Verification items for the finished model (mm, model axes). A direction names the side the tool comes from. Give positions to 0.01 mm unless a question says otherwise; leave off trailing zeros. Loops run counter-clockwise (first coordinate to the right, second up) from the corner with the lowest first, then second, coordinate; pieces in that order, holes last. Notation, with made-up numbers: (58, -26.5) - (101, -26.5) arc R15 cw to (101, 2.5) - close; hole circle Ø2 at (87.25, -28.75). An arc over 180 degrees is marked (long way). Use one line per item in the form item = value.
```python
from build123d import *

# Parameters (mm, degrees)
SKETCH1_W           = 5.6
SKETCH1_H           = 5.6
BOSS_EXTRUDE1_DEPTH = 1
SKETCH1_3_R         = 1.85
BOSS_EXTRUDE2_DEPTH = 11.7
SKETCH2_R           = 0.6
CUT_EXTRUDE1_DEPTH  = 5
BOSS_EXTRUDE3_START = 2
SKETCH3_R           = 2.25
SKETCH3_R_2         = 0.6
BOSS_EXTRUDE3_DEPTH = 2
CHAMFER1_SIZE       = 1.5
CHAMFER1_SIZE2      = 0.401923789
SKETCH4_W           = 1
SKETCH4_H           = 5.286883196
CUT_EXTRUDE3_DEPTH  = 4
FILLET1_R           = 1.5


with BuildPart() as part:
    # Sketch1 → Boss-Extrude1 (new body)
    with BuildSketch(Plane.XY):
        Rectangle(SKETCH1_W, SKETCH1_H)
    extrude(amount=BOSS_EXTRUDE1_DEPTH)

    # Sketch1<3> → Boss-Extrude2 (add)
    with BuildSketch(Plane.XY):
        Circle(SKETCH1_3_R)
    extrude(amount=-BOSS_EXTRUDE2_DEPTH)

    # Sketch2 → Cut-Extrude1 (cut)
    with BuildSketch(Plane(origin=(0, 0, -11.7), x_dir=(-1, 0, 0), z_dir=(0, 0, -1))):
        Circle(SKETCH2_R)
    extrude(amount=-CUT_EXTRUDE1_DEPTH, mode=Mode.SUBTRACT)

    # Sketch3 → Boss-Extrude3 (add)
    with BuildSketch(Plane(origin=(0, 0, -11.7), x_dir=(-1, 0, 0), z_dir=(0, 0, -1)).offset(BOSS_EXTRUDE3_START)):
        Circle(SKETCH3_R)
        Circle(SKETCH3_R_2, mode=Mode.SUBTRACT)
    extrude(amount=-BOSS_EXTRUDE3_DEPTH)

    # Chamfer1
    chamfer1_edges = [part.edges().sort_by_distance(p)[0] for p in [
        (2.25, 0, -13.7),
    ]]
    chamfer1_side = [part.faces().sort_by_distance(p)[0] for p in [
        (2.25, 0, -12.7),
    ]]
    chamfer(chamfer1_edges, length=CHAMFER1_SIZE, length2=CHAMFER1_SIZE2, reference=chamfer1_side[0])

    # Sketch4 → Cut-Extrude3 (cut)
    with BuildSketch(Plane(origin=(0, 0, -13.7), x_dir=(-1, 0, 0), z_dir=(0, 0, -1))):
        Rectangle(SKETCH4_W, SKETCH4_H)
    extrude(amount=-CUT_EXTRUDE3_DEPTH, mode=Mode.SUBTRACT)

    # Fillet1
    fillet1_edges = [part.edges().sort_by_distance(p)[0] for p in [
        (2.25, 0, -12.2),
        (-2.25, 0, -12.2),
    ]]
    fillet(fillet1_edges, radius=FILLET1_R)


solid = part.part
```
1. Section check A-A, the plane x = 0. Record the cut outline in (y, z).
Result set:
outline = (-2.8, 0) - (-1.85, 0) - (-1.85, -9.7) - (-0.6, -9.7) - (-0.6, -6.7) - (0.6, -6.7) - (0.6, -9.7) - (1.85, -9.7) - (1.85, 0) - (2.8, 0) - (2.8, 1) - (-2.8, 1) - close
2. Section check C-C, the plane y = 2.5. Record the cut outline in (x, z), then the cut area to 3 significant figures.
Result set:
outline = (-2.8, 0) - (2.8, 0) - (2.8, 1) - (-2.8, 1) - close
area = 5.60 mm²
3. Depth check by flat-ended pin: pin 1 Ø2 at (y, z) = (-1, -11) entering from +X; pin 2 Ø1 at (y, z) = (0, -6.5) entering from +X; pin 3 Ø1.5 at (x, z) = (0, -1.5) entering from -Y. Enter the tip coordinate at first touch or a pass-through.
Result set:
pin_1 = 2.23
pin_2 = 1.85
pin_3 = -1.85
4. Section check D-D, the plane z = -1.5. Record the cut outline in (x, y).
Result set:
outline = circle Ø3.7 at (0, 0)
5. Scan lines: probe 1 along Y at (x, z) = (0, -9.5); probe 2 along Z at (x, y) = (2.4, -0.25); probe 3 along Z at (x, y) = (0.4, 0.9). Record each from-to range of solid material in increasing order.
Result set:
probe_1 = -1.85 to -0.6, 0.6 to 1.85
probe_2 = 0 to 1
probe_3 = -9.7 to 1
6. Section check B-B, the plane z = -9.5. Record the cut outline in (x, y).
Result set:
outline = circle Ø3.7 at (0, 0); hole circle Ø1.2 at (0, 0)
7. Draft check along X on faces 5 (the cylindrical face through (2.25, 0.04, -11.85)), 6 (the flat face through (0, 2.8, 0.5)), 7 (the cylindrical face through (-0.554, -0.23, -9.471)). Enter one of: released by +X, released by -X, zero draft, split by the parting line, or undercut.
Result set:
face_5 = released by +X
face_6 = zero draft
face_7 = undercut
8. Tool access check on faces 1 (the flat face through (2, -0.2, -11.7)), 2 (the cylindrical face through (-2.25, -0.04, -11.85)), 3 (the flat face through (-1, 2, 0)), 4 (the flat face through (0.5, -1, -12)). Record the directions out of +Z, -Z, +X, -X, +Y, -Y that give a thin tool (end or side, any length) a straight path to the whole face; none if there is none.
Result set:
face_1 = +X
face_2 = -Z, -X
face_3 = none
face_4 = -Z, +Y, -Y
